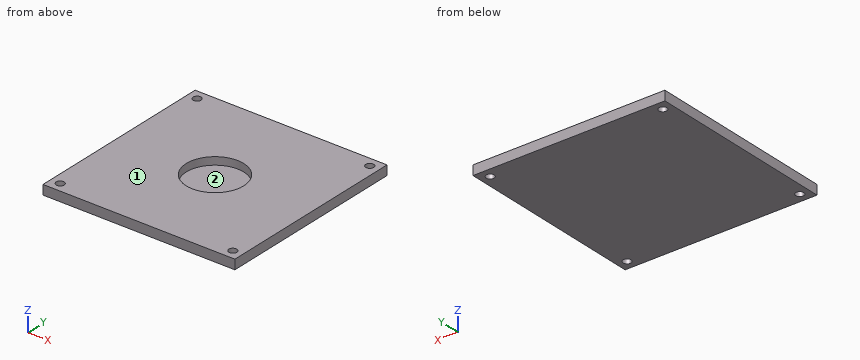
```python
from build123d import *

# Parameters (mm, degrees)
F0_W     = 100
F0_H     = 100
F0_R     = 2.1
F1_DEPTH = 5
F2_R     = 15
F3_DEPTH = 4


with BuildPart() as f1:
    # F0 (on Top) → F1 (new body)
    with BuildSketch(Plane.XY):
        with Locations((3.806381, 10.591754)):
            Rectangle(F0_W, F0_H)
        with Locations((-41.193619, -34.408246)):
            Circle(F0_R, mode=Mode.SUBTRACT)
        with Locations((48.806381, -34.408246)):
            Circle(F0_R, mode=Mode.SUBTRACT)
        with Locations((-41.193619, 55.591754)):
            Circle(F0_R, mode=Mode.SUBTRACT)
        with Locations((48.806381, 55.591754)):
            Circle(F0_R, mode=Mode.SUBTRACT)
    extrude(amount=F1_DEPTH)

    # F2 (on face) → F3 (cut)
    with BuildSketch(Plane.XY.offset(5)):
        with Locations((3.806381, 10.591754)):
            Circle(F2_R)
    extrude(amount=-F3_DEPTH, mode=Mode.SUBTRACT)


solid = f1.part
```
Check sheet for the modelled part. Datum: model origin and axes. Units: mm. Face numbers are marked on the shaded views. Give positions to 0.01 mm unless a question says otherwise; leave off trailing zeros. Order: outer loops, then holes, each group sorted by start corner. A loop starts at its lowest first (then second) coordinate and runs counter-clockwise, first axis right, second up. Notation, with made-up numbers: (78, 74) -> (85, 74) arc R18 ccw to (85, 82) -> close; hole circle Ø8 at (75.5, 7). An arc over 180 degrees is marked (long way). Use CSV: the item, a comma, the result in double quotes. Start each with the question number.
1) Sectioned sample at C-C, the plane y = 9. Record the boundary of the cut face in (x, z).
2) Sectioned sample at B-B, the plane z = 3.6. Record the boundary of the cut face in (x, y).
3) Sectioned sample at A-A, the plane x = 1. Record the boundary of the cut face in (y, z).
4) Go/stop test with a flat-tipped pin: P1, Ø18, axis at x = 3.81, y = 10.59, coming from the +Z side. Record where the tip stops, or that it passes through.
5) Material ranges on line 1 (Y direction, x = -41.5, z = 0.65); line 2 (X direction, y = 13.5, z = 1.05); line 3 (X direction, y = 56, z = 4.85), recorded low to high. Write a range as from..to.
6) Mould release check, pull along Y, two halves, no side actions. Record for the marked faces 1 and 2: released by +Y, released by -Y, zero draft, split by the parting line, or undercut.
Recorded:
1,outline,"(-46.19, 0) -> (53.81, 0) -> (53.81, 5) -> (18.72, 5) -> (18.72, 1) -> (-11.11, 1) -> (-11.11, 5) -> (-46.19, 5) -> close"
2,outline,"(-46.19, -39.41) -> (53.81, -39.41) -> (53.81, 60.59) -> (-46.19, 60.59) -> close; hole circle Ø4.2 at (-41.19, -34.41); hole circle Ø4.2 at (-41.19, 55.59); hole circle Ø30 at (3.81, 10.59); hole circle Ø4.2 at (48.81, -34.41); hole circle Ø4.2 at (48.81, 55.59)"
3,outline,"(-39.41, 0) -> (60.59, 0) -> (60.59, 5) -> (25.33, 5) -> (25.33, 1) -> (-4.14, 1) -> (-4.14, 5) -> (-39.41, 5) -> close"
4,P1,"z = 1"
5,line 1,"-39.41..-36.49, -32.33..53.51, 57.67..60.59"
5,line 2,"-46.19..-10.91, 18.52..53.81"
5,line 3,"-46.19..-43.25, -39.13..46.75, 50.87..53.81"
6,face 1,"zero draft"
6,face 2,"undercut"
